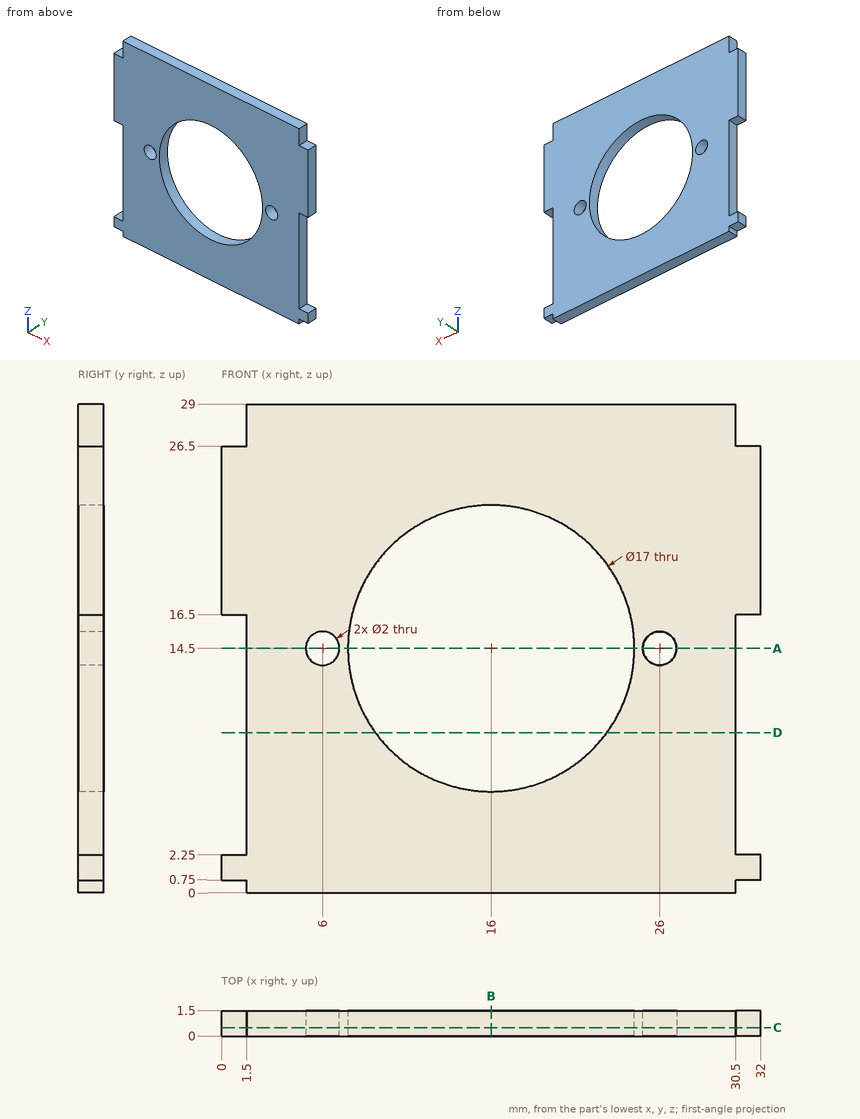
Geometry: see drawing. Coordinates: mm, zero at the bounding-box minimum. Coordinates: 2 decimals unless noted, no trailing zeros. Order: outer loops, then holes, each group sorted by start corner. A loop starts at its lowest first (then second) coordinate and runs counter-clockwise, first axis right, second up. Notation, with made-up numbers: M 6.25,80.25 L 59.25,80.25 A22 ccw 59.25,112.25 Z; hole C 61,71.5 d6. An arc over 180 degrees is marked long. Answer in a Markdown table with one row per item. Add a question column.
Q1. Contact query for flat-ended pins moving along their axis: P1, Ø0.8, axis at y = 1, z = 0.5, coming from the +X side; P2, Ø1.6, axis at x = 26, z = 14.5, coming from the +Y side; P3, Ø0.6, axis at y = 1, z = 0, coming from the -X side. Output: stop coordinate, or through.
Q2. Section query C-C on y = 0.5. Return the cut outline in (x, z), and give its area (3 significant figures).
Q3. Section query D-D on z = 9.5. Return the cut outline in (x, y).
Q4. Section query A-A on z = 14.5. Return the cut outline in (x, y), and give its area (3 significant figures).
Q5. Section query B-B on x = 16. Return the cut outline in (y, z).
Q6. Line query: L1, parallel to Z at x = 16, y = 1.1; L2, parallel to X at y = 0.6, z = 13.75; L3, parallel to Z at x = 10, y = 0.65. Output: solid intervals per line, ascending.
Completed:
| question | item | result |
|---|---|---|
| 1 | P1 | stops at x = 32 |
| 1 | P2 | passes through |
| 1 | P3 | stops at x = 1.5 |
| 2 | outline | M 0,0.75 L 1.5,0.75 L 1.5,0 L 30.5,0 L 30.5,0.75 L 32,0.75 L 32,2.25 L 30.5,2.25 L 30.5,16.5 L 32,16.5 L 32,26.5 L 30.5,26.5 L 30.5,29 L 1.5,29 L 1.5,26.5 L 0,26.5 L 0,16.5 L 1.5,16.5 L 1.5,2.25 L 0,2.25 Z; hole C 6,14.5 d2; hole C 16,14.5 d17; hole C 26,14.5 d2 |
| 2 | area | 642 mm2 |
| 3 | outline | M 1.5,0 L 9.13,0 L 9.13,1.5 L 1.5,1.5 Z; M 22.87,0 L 30.5,0 L 30.5,1.5 L 22.87,1.5 Z |
| 4 | outline | M 1.5,0 L 5,0 L 5,1.5 L 1.5,1.5 Z; M 7,0 L 7.5,0 L 7.5,1.5 L 7,1.5 Z; M 24.5,0 L 25,0 L 25,1.5 L 24.5,1.5 Z; M 27,0 L 30.5,0 L 30.5,1.5 L 27,1.5 Z |
| 4 | area | 12.0 mm2 |
| 5 | outline | M 0,0 L 1.5,0 L 1.5,6 L 0,6 Z; M 0,23 L 1.5,23 L 1.5,29 L 0,29 Z |
| 6 | L1 | z = 0 to 6, 23 to 29 |
| 6 | L2 | x = 1.5 to 5.34, 6.66 to 7.53, 24.47 to 25.34, 26.66 to 30.5 |
| 6 | L3 | z = 0 to 8.48, 20.52 to 29 |
